Part print with two shaded views. Sizes in mm from the minimum x, y, z corner. A direction names the side the tool comes from. Round coordinates to 2 decimals unless told otherwise and drop trailing zeros. Loops run counter-clockwise (first coordinate to the right, second up) from the corner with the lowest first, then second, coordinate; pieces in that order, holes last. Notation, with made-up numbers: M -2,13 L 32,13 A20 ccw 32,49 Z; hole C 63,-30.5 d10. An arc over 180 degrees is marked long. Answer as CSV lines item,"result". Start each with the question number.
Item 1: Mould opens along X. For the marked faces 3, 4 and 5 say: pulls with the +X half, pulls with the -X half, needs draft (parallel to the pull), parting line crosses it, or undercut.
Item 2: Band-saw the part on C-C (x = 6.5). Give the cut face in (y, z).
Item 3: Wall check: line 1 (Y direction, x = 17.5, z = 2.25); line 2 (X direction, y = 8.25, z = 11); line 3 (Z direction, x = 10, y = 1.25) (1 decimal). Give the ranges that are in metal, low to high.
Item 4: Drop flat-ended pins along their axis: pin 1 Ø3.5 at (x, z) = (5.38, 16.62) entering from +Y; pin 2 Ø1.5 at (y, z) = (9.5, 14) entering from +X (1 decimal); pin 3 Ø9 at (x, z) = (11, 11) entering from +Y; pin 4 Ø5 at (y, z) = (8.5, 16.5) entering from -X. Give the stop position or say it passes through.
Item 5: Band-saw the part on A-A (x = 11). Give the cut face in (y, z), and give its area (3 significant figures).
Item 6: Band-saw the part on B-B (z = 11). Give the cut face in (x, y), and give its area (3 significant figures).
Item 7: Which spindle directions (+Z, -Z, +X, -X, +Y, -Y) get a long thin tool onto all of the face, cutting with end or side? Do the marked faces 1 and 2. Say none if no direction does.
Item 8: Band-saw the part on D-D (y = 10.25). Give the cut face in (x, z).
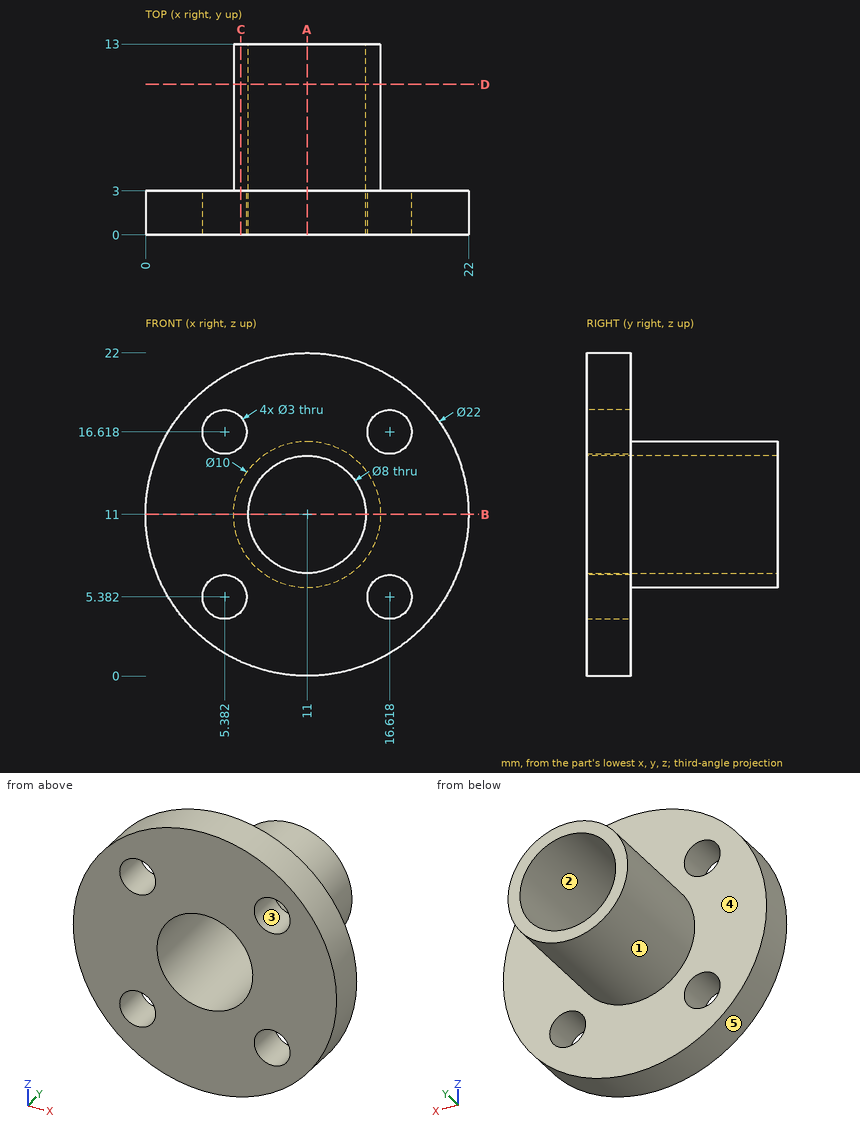
Answer block:
1,face 3,"undercut"
1,face 4,"needs draft"
1,face 5,"parting line crosses it"
2,outline,"M 0,0.96 L 3,0.96 L 3,4.38 L 0,4.38 Z; M 0,6.38 L 3,6.38 L 3,8.82 L 13,8.82 L 13,13.18 L 3,13.18 L 3,15.62 L 0,15.62 Z; M 0,17.62 L 3,17.62 L 3,21.04 L 0,21.04 Z"
3,line 1,"y = 0 to 3"
3,line 2,"x = 6 to 7, 15 to 16"
3,line 3,"z = 0 to 7.1, 14.9 to 22"
4,pin 1,"stops at y = 3"
4,pin 2,"stops at x = 15.5"
4,pin 3,"stops at y = 13"
4,pin 4,"stops at x = 7"
5,outline,"M 0,0 L 3,0 L 3,6 L 13,6 L 13,7 L 0,7 Z; M 0,15 L 13,15 L 13,16 L 3,16 L 3,22 L 0,22 Z"
5,area,"62.0 mm^2"
6,outline,"M 0,0 L 7,0 L 7,13 L 6,13 L 6,3 L 0,3 Z; M 15,0 L 22,0 L 22,3 L 16,3 L 16,13 L 15,13 Z"
6,area,"62.0 mm^2"
7,face 1,"+Y"
7,face 2,"+Y, -Y"
8,outline,"C 11,11 d10; hole C 11,11 d8"
